Autodesk Inventor part; units mm, degrees
ref_plane "YZ Plane" through (0, 0, 0) normal (1, 0, 0) x (0, 1, 0)
ref_plane "XZ Plane" through (0, 0, 0) normal (0, 1, 0) x (-1, 0, 0)
ref_plane "XY Plane" through (0, 0, 0) normal (0, 0, 1) x (1, 0, 0)
sketch "Sketch1" plane through (0, 0, 0) normal (0, 1, 0) x (-1, 0, 0)
  line L0 (0, 0) -> (125, 0)
  line L1 (125, 0) -> (125, -50)
  line L2 (125, -50) -> (0, -50)
  line L3 (0, -50) -> (0, 0)
  line L4 (0, 0) -> (0, -16.6667)
  line L5 (0, -16.6667) -> (6, -16.6667)
  line L6 (125, -50) -> (50, -50)
  line L7 (50, -50) -> (50, -110)
  line L8 (50, -110) -> (125, -110)
  line L9 (125, -110) -> (125, -50)
  point P0 (50, -50)
  dimension "d0" = 125
  dimension "d1" = 50
  dimension "d2" = 16.6667
  dimension "d3" = 6
  dimension "d90" = 75
  dimension "d91" = 60
extrude "Extrusion1" add sketch "Sketch1" along normal blind 6
sketch "Sketch3" plane through (0, 6, 0) normal (0, 1, 0) x (1, 0, 0)
  circle A0 centre (-13, 12.5) radius 2.75
  line L0 (0, 0) -> (0, 50)
  line L1 (-125, 0) -> (0, 0)
  circle A1 centre (-13, 37.5) radius 2.75
  line L2 (-13, 12.5) -> (-18, 12.5)
  line L3 (-23, 12.5) -> (-13, 12.5) construction
  line L4 (-23, 9.75) -> (-13, 9.75)
  line L5 (-13, 15.25) -> (-23, 15.25)
  arc A2 (-23, 15.25) -> (-23, 9.75) centre (-23, 12.5) ccw
  arc A3 (-13, 9.75) -> (-13, 15.25) centre (-13, 12.5) ccw
  line L6 (-13, 37.5) -> (-18, 37.5)
  line L7 (-13, 37.5) -> (-8, 37.5) construction
  line L8 (-23, 37.5) -> (-13, 37.5) construction
  line L9 (-23, 34.75) -> (-13, 34.75)
  line L10 (-13, 40.25) -> (-23, 40.25)
  arc A4 (-23, 40.25) -> (-23, 34.75) centre (-23, 37.5) ccw
  arc A5 (-13, 34.75) -> (-13, 40.25) centre (-13, 37.5) ccw
  dimension "d21" = 5.5
  dimension "d22" = 13
  dimension "d23" = 12.5
  dimension "d26" = 25
  dimension "d87" = 5
  dimension "d88" = 5
  dimension "d89" = 180
extrude "Extrusion3" cut sketch "Sketch3" against normal through all
sketch "Sketch4" plane through (0, 6, 0) normal (0, 1, 0) x (1, 0, 0)
  arc A0 (-13, 9.75) -> (-13, 15.25) centre (-13, 12.5) ccw
  line L0 (-13, 12.5) -> (-73, 12.5)
  line L1 (-73, 12.5) -> (-91, 12.5) construction
  line L2 (-73, 15.25) -> (-91, 15.25)
  line L3 (-91, 9.75) -> (-73, 9.75)
  arc A1 (-73, 9.75) -> (-73, 15.25) centre (-73, 12.5) ccw
  arc A2 (-91, 15.25) -> (-91, 9.75) centre (-91, 12.5) ccw
  point P0 (0, 0)
  point P1 (-82, 12.5)
  dimension "d33" = 60
  dimension "d34" = 18
  dimension "d35" = 5.5
extrude "Extrusion4" cut sketch "Sketch4" against normal through all
pattern_linear "Rectangular Pattern2" count 2 spacing 25 along (0, 0, -1) of "Extrusion4"
sketch "Sketch5" plane through (0, 0, -50) normal (0, 0, -1) x (-1, 0, 0)
  line L0 (125, 0) -> (125, 6)
  line L1 (125, 0) -> (0, 0)
  line L2 (125, 6) -> (100, 6)
  line L3 (100, 6) -> (100, 0)
  line L4 (100, 0) -> (125, 0)
  line L5 (125, 0) -> (125, 6)
  dimension "d45" = 25
fillet "Fillet2" radius 5 3 edges at (-125, 3, 0) (0, 3, 0) (0, 3, -50)
sketch "Sketch7" plane through (0, 6, 0) normal (0, 1, 0) x (1, 0, 0)
  arc A0 (-13, 9.75) -> (-13, 15.25) centre (-13, 12.5) ccw
  line L0 (-13, 12.5) -> (-35, 12.5)
  line L1 (-35, 12.5) -> (-55, 12.5)
  circle A1 centre (-55, 12.5) radius 2.75
  circle A2 centre (-35, 12.5) radius 2.75
  line L2 (0, 5) -> (0, 45)
  line L3 (0, 0) -> (0, 45)
  circle A3 centre (-35, 37.5) radius 2.75
  circle A4 centre (-55, 37.5) radius 2.75
  dimension "d55" = 22
  dimension "d56" = 20
  dimension "d57" = 5.5
  dimension "d58" = 5.5
  dimension "d61" = 25
extrude "Extrusion7" cut sketch "Sketch7" against normal through all
sketch "Sketch9" plane through (0, 6, 0) normal (0, 1, 0) x (1, 0, 0)
  point P0 (0, 0)
sketch "Sketch12" plane through (0, 6, 0) normal (0, 1, 0) x (1, 0, 0)
  line L0 (-50, 110) -> (-125, 110)
  circle A0 centre (-73, 100) radius 3
  line L1 (-73, 100) -> (-73, 60)
  circle A1 centre (-73, 60) radius 3
  line L2 (-125, 110) -> (-125, 5)
  line L3 (-50, 50) -> (-50, 110)
  arc A2 (-73, 34.75) -> (-73, 40.25) centre (-73, 37.5) ccw
  line L4 (-73, 100) -> (-113, 100)
  circle A3 centre (-113, 100) radius 3
  point P0 (0, 0)
  dimension "d93" = 6
  dimension "d94" = 40
  dimension "d96" = 6
  dimension "d102" = 0
  dimension "d103" = 10
  dimension "d104" = 40
  dimension "d105" = 6
extrude "Extrusion10" cut sketch "Sketch12" against normal through all
fillet "Fillet3" radius 5 2 edges at (-125, 3, -110) (-50, 3, -110)
fillet "Fillet4" radius 5 1 edges at (-50, 3, -50)
sketch "Sketch13" plane through (0, 6, 0) normal (0, 1, 0) x (1, 0, 0)
  circle A0 centre (-113, 100) radius 3
  circle A1 centre (-113, 100) radius 20
  circle A2 centre (-113, 100) radius 37
  circle A3 centre (-73, 100) radius 3
  line L0 (-113, 100) -> (-133, 100)
  line L1 (-133, 100) -> (-150, 100)
  line L2 (-133, 100) -> (-116, 100) construction
  line L3 (-113, 100) -> (-77.377, 110)
  line L4 (-55, 110) -> (-120, 110)
  line L5 (-113, 100) -> (-93.7443, 105.4054)
  point P0 (0, 0)
  point P1 (-95.6795, 110)
  point P2 (-110.1116, 100.8108)
  dimension "d108" = 40
  dimension "d109" = 17
  dimension "d110" = 180
extrude "Extrusion11" add sketch "Sketch13" against normal blind 6 contours A0 L0 A1 L3 | L1 A2 L4 A1 picked at (-127.1454, 101.5717)
sketch "Sketch14" plane through (0, 6, 0) normal (0, 1, 0) x (1, 0, 0)
  circle A0 centre (-113, 100) radius 3
  arc A1 (-103, 117.3205) -> (-131.7939, 106.8404) centre (-113, 100) ccw construction
  arc A2 (-101.5, 119.9186) -> (-134.6129, 107.8665) centre (-113, 100) ccw
  arc A3 (-104.5, 114.7224) -> (-128.9748, 105.8143) centre (-113, 100) ccw
  arc A4 (-104.5, 114.7224) -> (-101.5, 119.9186) centre (-103, 117.3205) ccw
  arc A5 (-134.6129, 107.8665) -> (-128.9748, 105.8143) centre (-131.7939, 106.8404) ccw
  line L0 (-113, 100) -> (-131.7939, 106.8404) construction
  line L1 (-113, 100) -> (-93, 100) construction
  line L2 (-113, 100) -> (-103, 117.3205) construction
  point P0 (0, 0)
  dimension "d113" = 20
  dimension "d114" = 160
  dimension "d115" = 100
  dimension "d116" = 6
extrude "Extrusion12" cut sketch "Sketch14" against normal through all contours A4 A3 A5 A2
fillet "Fillet5" radius 5 2 edges at (-150, 3, -100) (-125, 3, -100)
fillet "Fillet6" radius 5 1 edges at (-77.377, 3, -110)
properties part number "CableChain_Plate"
Here's how the part is built. I have some questions about the finished solid (model axes, mm). A direction names the side the tool comes from. Coordinates: 2 decimals unless noted, no trailing zeros. Loops run counter-clockwise (first coordinate to the right, second up) from the corner with the lowest first, then second, coordinate; pieces in that order, holes last. Notation, with made-up numbers: (-22.75, 61.5) -> (15.25, 61.5) arc R19 cw to (15.25, 72.5) -> close; hole circle Ø3 at (33.25, -18.5). An arc over 180 degrees is marked (long way). Use one line per item in the form item = value. Start each with the question number.
(1) If we section it at A-A (z = -60): Please give me the cut outline in (x, y), then the cut area to 3 significant figures.
(2) Will these pins go through, and if not, where does the flat tip stop? pin 1 (3 mm diameter, centred on y = 2, z = -75.5, fed in from +X); pin 2 (3 mm diameter, centred on y = 3.5, z = -35, fed in from -X); pin 3 (1 mm diameter, centred on x = -43.5, y = 3.5, fed in from -Z).
(3) We'd pull the mould along X, two halves only. Please class faces 4 (the face through (-25.75, 3.04, -37.56)), 5 (the face through (-1, 3, -48)), 6 (the face through (-137, 3, -100)): pulls with the +X half, pulls with the -X half, needs draft (parallel to the pull), parting line crosses it, or undercut.
(4) If we section it at D-D (y = 3.6): Give the number of separate pieces and of enclosed holes in the cut face, then the cut area to 3 significant figures.
(5) On a 3-axis mill with a long thin cutter (end or side, diameter ignored), from which of +Z, -Z, +X, -X, +Y, -Y can I reach the whole of each face in a straight line? I mean faces 1 (the face through (-90, 6, -52)), 2 (the face through (-18, 3, -9.75)), 3 (the face through (-64, 3, -110)). Say none if no direction works.
(6) Please list where these lines run through material, in increasing order: line 1 along Z through (x, y) = (-35, 2.85); line 2 along Z through (x, y) = (-84, 5.25); line 3 along X through (y, z) = (4.5, -12.5).
(7) If we section it at C-C (z = -37.5): Please give me the cut outline in (x, y), then the cut area to 3 significant figures.
(8) If we section it at B-B (x = -113): Please give me the cut outline in (y, z), then the cut area to 3 significant figures.
Verdict:
q1.outline = (-125, 0) -> (-76, 0) -> (-76, 6) -> (-125, 6) -> close; (-70, 0) -> (-50, 0) -> (-50, 6) -> (-70, 6) -> close
q1.area = 414 mm²
q2.pin_1 = -50
q2.pin_2 = -125
q2.pin_3 = -50
q3.face_4 = undercut
q3.face_5 = pulls with the +X half
q3.face_6 = needs draft
q4.separate_pieces = 1
q4.enclosed_holes = 12
q4.area = 11,600 mm²
q5.face_1 = +Z, -Z, +X, -X, +Y
q5.face_2 = +Y, -Y
q5.face_3 = -Z, +X, +Y, -Y
q6.line_1 = -50 to -40.25, -34.75 to -15.25, -9.75 to 0
q6.line_2 = -122.98 to -40.25, -34.75 to -15.25, -9.75 to 0
q6.line_3 = -125 to -93.75, -70.25 to -57.75, -52.25 to -37.75, -32.25 to -25.75, -10.25 to 0
q7.outline = (-125, 0) -> (-93.75, 0) -> (-93.75, 6) -> (-125, 6) -> close; (-70.25, 0) -> (-57.75, 0) -> (-57.75, 6) -> (-70.25, 6) -> close; (-52.25, 0) -> (-37.75, 0) -> (-37.75, 6) -> (-52.25, 6) -> close; (-32.25, 0) -> (-25.75, 0) -> (-25.75, 6) -> (-32.25, 6) -> close; (-10.25, 0) -> (0, 0) -> (0, 6) -> (-10.25, 6) -> close
q7.area = 450 mm²
q8.outline = (0, -137) -> (6, -137) -> (6, -123) -> (0, -123) -> close; (0, -117) -> (6, -117) -> (6, -103) -> (0, -103) -> close; (0, -97) -> (6, -97) -> (6, 0) -> (0, 0) -> close
q8.area = 750 mm²
